Source: CAD feature listing. Evaluate the final solid. Frame: model axes, mm. Coordinates: 2 decimals unless noted, no trailing zeros. Write each loop counter-clockwise with the first axis right and the second up, starting at its lowest first coordinate (ties: lowest second). Pieces come first, ordered by that corner, then holes. Notation, with made-up numbers: M 66.5,40 L 94.5,40 A14 cw 94.5,61 Z; hole C 53.25,-18 d4. An arc over 180 degrees is marked long. One line per item, written item: value. Start each with the question number.
Item 1: Ray query, L1, parallel to X at y = -4.75, z = 98.5 (3 decimals). Return the intervals inside material, ascending. Write a range as from..to.
Item 2: Pin query (flat end, axial travel): P1, Ø7.5, axis at x = 0, z = 305.51, coming from the -Y side; P2, Ø5, axis at x = 0, z = -304.8, coming from the -Y side. Return the tip coordinate at first contact, or that it passes through.
Item 3: Cut plane B-B, the plane y = -1.5. Output: boundary loops of the cut face in (x, z) (3 decimals), then the cut area to 3 significant figures.
Item 4: Cut plane A-A, the plane z = -199. Output: boundary loops of the cut face in (x, y) (3 decimals).
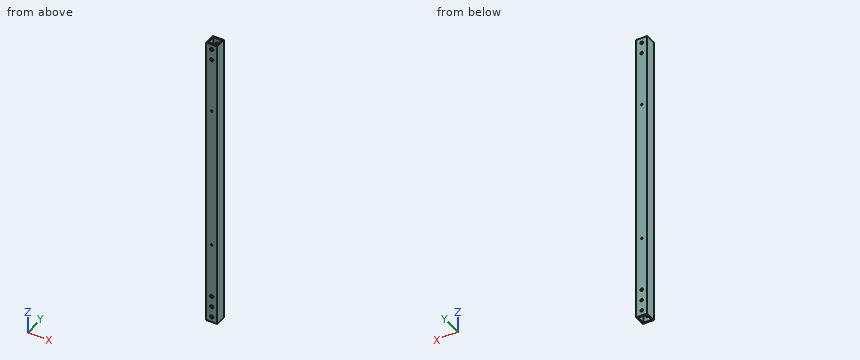
```python
from build123d import *

# Parameters (mm, degrees)
BOSS_EXTRUDE1_DEPTH                  = 342.9
BOSS_EXTRUDE1_DEPTH_BACK             = 342.9
SKETCH3_W                            = 25.4
SKETCH3_H                            = 25.4
SKETCH3_W_2                          = 19.05
SKETCH3_H_2                          = 19.05
F_5_32_0_15625_DIAMETER_HOLE1_D      = 3.96875
F_1_4_0_25_DIAMETER_HOLE1_AT_2_COUNT = 2
F_1_4_0_25_DIAMETER_HOLE1_AT_2_PITCH = 25.4
F_1_4_0_25_DIAMETER_HOLE1_AT_3_COUNT = 2
F_1_4_0_25_DIAMETER_HOLE1_AT_3_PITCH = 50.8
F_1_4_0_25_DIAMETER_HOLE2_AT_2_COUNT = 2
F_1_4_0_25_DIAMETER_HOLE2_AT_2_PITCH = 25.4


with BuildPart() as part:
    # Sketch3 → Boss-Extrude1 (new, two sides: drawn at the far end of the back side and taken through both)
    with BuildSketch(Plane.XY.offset(-BOSS_EXTRUDE1_DEPTH_BACK)):
        Rectangle(SKETCH3_W, SKETCH3_H)
        Rectangle(SKETCH3_W_2, SKETCH3_H_2, mode=Mode.SUBTRACT)
    extrude(amount=BOSS_EXTRUDE1_DEPTH + BOSS_EXTRUDE1_DEPTH_BACK)

    # 5/32 (0.15625) Diameter Hole1 (through all)
    with Locations(Plane(origin=(0, 12.7, 0), x_dir=(1, 0, 0), z_dir=(0, 1, 0))):
        with Locations((0, 152.4), (0, -178.5118096)):
            Hole(F_5_32_0_15625_DIAMETER_HOLE1_D / 2)

    # Sketch9 → 1/4 (0.25) Diameter Hole1 (revolve, cut)
    with BuildSketch(Plane(origin=(0, 12.7, -330.2), x_dir=(0, 0, 1), z_dir=(1, 0, 0))):
        Polygon((0, 0), (0, 25.4), (3.9624, 25.4), (3.175, 24.494199916), (3.175, 0), align=None)
    f_1_4_0_25_diameter_hole1 = revolve(axis=Axis((0, 19.05, -330.2), (0, -1, 0)), mode=Mode.SUBTRACT)

    # 1/4 (0.25) Diameter Hole1 at 2: 1/4 (0.25) Diameter Hole1 ×2
    with Locations(*[(0, 0, i * F_1_4_0_25_DIAMETER_HOLE1_AT_2_PITCH) for i in range(1, F_1_4_0_25_DIAMETER_HOLE1_AT_2_COUNT)]):
        add(f_1_4_0_25_diameter_hole1, mode=Mode.SUBTRACT)

    # 1/4 (0.25) Diameter Hole1 at 3: 1/4 (0.25) Diameter Hole1 ×2
    with Locations(*[(0, 0, i * F_1_4_0_25_DIAMETER_HOLE1_AT_3_PITCH) for i in range(1, F_1_4_0_25_DIAMETER_HOLE1_AT_3_COUNT)]):
        add(f_1_4_0_25_diameter_hole1, mode=Mode.SUBTRACT)

    # Sketch12 → 1/4 (0.25) Diameter Hole2 (revolve, cut)
    with BuildSketch(Plane(origin=(0, 12.7, 330.911799988), x_dir=(0, 0, 1), z_dir=(1, 0, 0))):
        Polygon((0, 0), (0, 25.4), (3.9624, 25.4), (3.175, 24.494199916), (3.175, 0), align=None)
    f_1_4_0_25_diameter_hole2 = revolve(axis=Axis((0, 19.05, 330.911799988), (0, -1, 0)), mode=Mode.SUBTRACT)

    # 1/4 (0.25) Diameter Hole2 at 2: 1/4 (0.25) Diameter Hole2 ×2
    with Locations(*[(0, 0, -i * F_1_4_0_25_DIAMETER_HOLE2_AT_2_PITCH) for i in range(1, F_1_4_0_25_DIAMETER_HOLE2_AT_2_COUNT)]):
        add(f_1_4_0_25_diameter_hole2, mode=Mode.SUBTRACT)


solid = part.part
```
From the geometry:
1. L1: x = -12.7..-9.525, 9.525..12.7
2. P1: stops at y = -12.46
2. P2: passes through
3. outline: M -12.7,-342.9 L -9.525,-342.9 L -9.525,342.9 L -12.7,342.9 Z; M 9.525,-342.9 L 12.7,-342.9 L 12.7,342.9 L 9.525,342.9 Z
3. area: 4,350 mm²
4. outline: M -12.7,-12.7 L 12.7,-12.7 L 12.7,12.7 L -12.7,12.7 Z; hole M -9.525,-9.525 L 9.525,-9.525 L 9.525,9.525 L -9.525,9.525 Z
